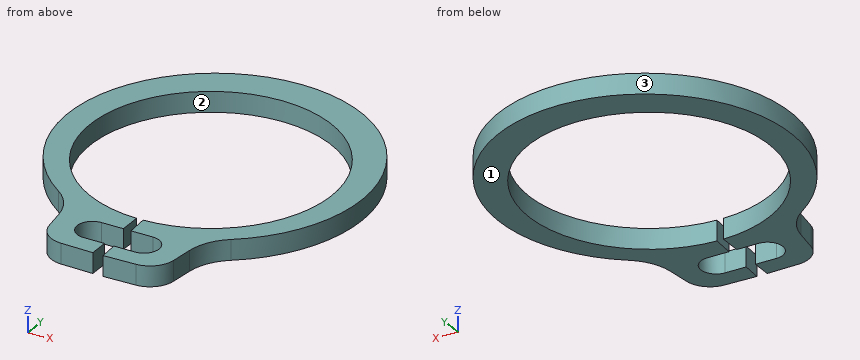
from build123d import *

# Parameters (mm, degrees)
BODYSKE_R   = 0.3
BODY_DEPTH  = 0.4
NOTSKE_W    = 1
NOTSKE_H    = 0.6
NOTCH_DEPTH = 1.4


with BuildPart() as part:
    # BodySke → Body (new body)
    with BuildSketch(Plane.XY):
        with BuildLine():
            Line((0.062913907, -2.374166557), (0.1, -3.773675264))
            Line((0.1, -3.773675264), (0.725313694, -3.757104848))
            ThreePointArc((0.725313694, -3.757104848), (1.046692153, -3.628800321), (1.207791092, -3.322543406))
            Line((1.207791092, -3.322543406), (1.26381232, -2.897019935))
            ThreePointArc((1.26381232, -2.897019935), (1.3982129, -2.512352239), (1.674947292, -2.213268924))
            ThreePointArc((1.674947292, -2.213268924), (0, 3.025), (-1.674947292, -2.213268924))
            ThreePointArc((-1.674947292, -2.213268924), (-1.3982129, -2.512352239), (-1.26381232, -2.897019935))
            Line((-1.26381232, -2.897019935), (-1.207791092, -3.322543406))
            ThreePointArc((-1.207791092, -3.322543406), (-1.046692153, -3.628800321), (-0.725313694, -3.757104848))
            Line((-0.725313694, -3.757104848), (-0.1, -3.773675264))
            Line((-0.1, -3.773675264), (-0.062913907, -2.374166557))
            ThreePointArc((-0.062913907, -2.374166557), (0, 2.375), (0.062913907, -2.374166557))
        make_face()
        with Locations((0.5, -3.097403146)):
            Circle(BODYSKE_R, mode=Mode.SUBTRACT)
        with Locations((-0.5, -3.097403146)):
            Circle(BODYSKE_R, mode=Mode.SUBTRACT)
    extrude(amount=-BODY_DEPTH)

    # NotSke → Notch (cut, through all)
    with BuildSketch(Plane.XY):
        with Locations((0, -3.097403146)):
            Rectangle(NOTSKE_W, NOTSKE_H)
    extrude(amount=-NOTCH_DEPTH, mode=Mode.SUBTRACT)


solid = part.part
Could you check a few things on this model? Use its own coordinates, in mm. Face numbers are marked on the shaded views. Give positions to 0.01 mm unless a question says otherwise; leave off trailing zeros. Write each loop counter-clockwise with the first axis right and the second up, starting at its lowest first coordinate (ties: lowest second). Pieces come first, ordered by that corner, then holes. Notation, with made-up numbers: (71, 52) -> (97, 52) arc R23 cw to (97, 72) -> close; hole circle Ø1 at (3.25, 40). An arc over 180 degrees is marked (long way). Answer as a JSON object with one key per item and string values.
Q1. We'd pull the mould along Y, two halves only. Please class the marked faces 1, 2 and 3: released by +Y, released by -Y, zero draft, split by the parting line, or undercut.
Taken from the geometry:
{"face 1": "zero draft", "face 2": "undercut", "face 3": "split by the parting line"}
Q2. Suppose I cut it at A-A on y = 1. Write out the boundary of the cut face in (x, z).
Taken from the geometry:
{"outline": "(-2.76, -0.4) -> (-2.15, -0.4) -> (-2.15, 0) -> (-2.76, 0) -> close; (2.15, -0.4) -> (2.76, -0.4) -> (2.76, 0) -> (2.15, 0) -> close"}
Q3. Please list where these lines run through material, in increasing order: L1, parallel to Y at x = -0.7, z = -0.3; L2, parallel to Y at x = 0.45, z = -0.1; L3, parallel to X at y = 0.25, z = -0.2.
Taken from the geometry:
{"L1": "y = -3.76 to -3.32, -2.87 to -2.27, 2.27 to 2.94", "L2": "y = -3.76 to -3.4, -2.8 to -2.33, 2.33 to 2.99", "L3": "x = -2.88 to -2.36, 2.36 to 2.88"}
Q4. Suppose I cut it at B-B on x = -1.55. Write out the boundary of the cut face in (y, z).
Taken from the geometry:
{"outline": "(-2.32, -0.4) -> (-1.8, -0.4) -> (-1.8, 0) -> (-2.32, 0) -> close; (1.8, -0.4) -> (2.57, -0.4) -> (2.57, 0) -> (1.8, 0) -> close"}
